Read the model definition and answer for the solid it produces. Units are mm, in the model's axes. A direction names the side the tool comes from. Give positions to 0.01 mm unless a question says otherwise; leave off trailing zeros. Loops run counter-clockwise (first coordinate to the right, second up) from the corner with the lowest first, then second, coordinate; pieces in that order, holes last.
(1) Find section B-B, the plane x = 26. Write down the section's boundary in (y, z), then the cut area to 3 significant figures.
(2) Which of the six approach directions +Z, -Z, +X, -X, +Y, -Y give full straight-line access (tool end or side, diameter ignored) to faces 1 (the face through (0, 197, 30)), 2 (the face through (0, 197, -30)), 3 (the face through (30, 197, 0))?
(3) Find section A-A, the plane z = 0. Write down the section's boundary in (x, y).
(4) Find section D-D, the plane y = 55. Write down the section's boundary in (x, z), then the cut area to 3 significant figures.
(5) Straight lines are drawn through the part: probe 1 along Y at (x, z) = (14.5, 44.5); probe 2 along Z at (x, y) = (-17, 66). For each, find the intervals that lie inside material, in ascending order.
(6) Find section C-C, the plane y = -5.5. Write down the section's boundary in (x, z).
(7) Each of these flat-tipped pins is pushed along its axis until it touches: P1, Ø1, axis at x = 3, y = 149.5, coming from the -Z side; P2, Ø8, axis at y = 206.5, z = 6, coming from the -X side; P3, Ø8, axis at y = 45, z = -26, coming from the +X side; P4, Ø2, axis at x = -31.5, y = 202, coming from the +Z side. Where does it stop, or does it pass through?
```python
from build123d import *

# Parameters (mm, degrees)
SKETCH_1_W      = 60
SKETCH_1_H      = 60
EXTRUDE_1_DEPTH = 400
SKETCH_2_R      = 50
EXTRUDE_2_DEPTH = 50


with BuildPart() as part:
    # 草图1 → 凸台-拉伸1 (new body)
    with BuildSketch(Plane(origin=(0, 0, 0), x_dir=(1, 0, 0), z_dir=(0, 1, 0))):
        Rectangle(SKETCH_1_W, SKETCH_1_H)
    extrude(amount=EXTRUDE_1_DEPTH)

    # 草图2 → 凸台-拉伸2 (add)
    with BuildSketch(Plane.XZ):
        with Locations(Location((0, 0, 0), (0, 0, 270))):
            Circle(SKETCH_2_R)
    extrude(amount=EXTRUDE_2_DEPTH)


solid = part.part
```
Entries:
1. outline: (-50, -42.71) - (0, -42.71) - (0, -30) - (400, -30) - (400, 30) - (0, 30) - (0, 42.71) - (-50, 42.71) - close
1. area: 28,300 mm2
2. face 1: +Z, +X, -X, +Y
2. face 2: -Z, +X, -X, +Y
2. face 3: +Z, -Z, +X, +Y
3. outline: (-50, -50) - (50, -50) - (50, 0) - (30, 0) - (30, 400) - (-30, 400) - (-30, 0) - (-50, 0) - close
4. outline: (-30, -30) - (30, -30) - (30, 30) - (-30, 30) - close
4. area: 3,600 mm2
5. probe 1: y = -50 to 0
5. probe 2: z = -30 to 30
6. outline: circle Ø100 at (0, 0)
7. P1: stops at z = -30
7. P2: stops at x = -30
7. P3: stops at x = 30
7. P4: passes through
